```python
from build123d import *

# Parameters (mm, degrees)
SKETCH1_R           = 30
SKETCH1_R_2         = 27.5
BOSS_EXTRUDE1_DEPTH = 100
SKETCH1_2_R         = 27.5
BOSS_EXTRUDE2_DEPTH = 5
SKETCH2_W           = 1.5
SKETCH2_H           = 49.5
BOSS_EXTRUDE3_DEPTH = 40
SKETCH3_W           = 42
SKETCH3_H           = 49.5
BOSS_EXTRUDE4_DEPTH = 2
BOSS_EXTRUDE5_DEPTH = 49.5


with BuildPart() as part:
    # Sketch1 → Boss-Extrude1 (new body)
    with BuildSketch(Plane(origin=(0, 0, 0), x_dir=(1, 0, 0), z_dir=(0, 1, 0))):
        with Locations(Location((0, 0, 0), (0, 0, 270))):
            Circle(SKETCH1_R)
        with Locations(Location((0, 0, 0), (0, 0, 270))):
            Circle(SKETCH1_R_2, mode=Mode.SUBTRACT)
    extrude(amount=BOSS_EXTRUDE1_DEPTH)

    # Sketch1<2> → Boss-Extrude2 (add)
    with BuildSketch(Plane(origin=(0, 0, 0), x_dir=(1, 0, 0), z_dir=(0, 1, 0))):
        with Locations(Location((0, 0, 0), (0, 0, 270))):
            Circle(SKETCH1_2_R)
    extrude(amount=BOSS_EXTRUDE2_DEPTH)

    # Sketch2 → Boss-Extrude3 (add)
    with BuildSketch(Plane.XZ):
        with Locations((-20.25, 0)):
            Rectangle(SKETCH2_W, SKETCH2_H)
        with Locations((20.25, 0)):
            Rectangle(SKETCH2_W, SKETCH2_H)
    extrude(amount=BOSS_EXTRUDE3_DEPTH)

    # Sketch3 → Boss-Extrude4 (add)
    with BuildSketch(Plane.XZ):
        Rectangle(SKETCH3_W, SKETCH3_H)
    extrude(amount=-BOSS_EXTRUDE4_DEPTH)

    # Sketch4 → Boss-Extrude5 (add)
    with BuildSketch(Plane(origin=(0, 0, -24.75), x_dir=(-1, 0, 0), z_dir=(0, 0, -1))):
        Polygon((21, -40), (22.5, -38.5), (21, -38.5), align=None)
        Polygon((-21, -40), (-22.5, -38.5), (-21, -38.5), align=None)
    extrude(amount=-BOSS_EXTRUDE5_DEPTH)


solid = part.part
```
CAD build for the part. Positions are in the model's coordinates, mm. A direction names the side the tool comes from. Give positions to 0.01 mm unless a question says otherwise; leave off trailing zeros. Loops run counter-clockwise (first coordinate to the right, second up) from the corner with the lowest first, then second, coordinate; pieces in that order, holes last. Notation, with made-up numbers: (34.5, 23.5) -> (74.5, 23.5) arc R13 ccw to (74.5, 28.5) -> close; hole circle Ø11 at (-12, 64). An arc over 180 degrees is marked (long way). Use a Markdown table: item, result.
1. Slice it at D-D (z = 0). List the corners of the cut face in (x, y).
Check result:
| item | result |
|---|---|
| outline | (-30, 0) -> (-21, 0) -> (-21, -38.5) -> (-22.5, -38.5) -> (-21, -40) -> (-19.5, -40) -> (-19.5, 0) -> (19.5, 0) -> (19.5, -40) -> (21, -40) -> (22.5, -38.5) -> (21, -38.5) -> (21, 0) -> (30, 0) -> (30, 100) -> (27.5, 100) -> (27.5, 5) -> (-27.5, 5) -> (-27.5, 100) -> (-30, 100) -> close |
2. Flat gauge pins, fed straight in: pin 1 (12 mm diameter, centred on y = -12.5, z = -1, fed in from +X); pin 2 (1 mm diameter, centred on x = 23.5, y = 55, fed in from -Z); pin 3 (10 mm diameter, centred on y = 28.5, z = -7, fed in from -X). Where does each tip first touch, or does it go through?
Check result:
| item | result |
|---|---|
| pin 1 | stops at x = 21 |
| pin 2 | stops at z = -19.26 |
| pin 3 | stops at x = -29.93 |
3. Slice it at B-B (z = 19). List the corners of the cut face in (x, y).
Check result:
| item | result |
|---|---|
| outline | (-23.22, 0) -> (-21, 0) -> (-21, -38.5) -> (-22.5, -38.5) -> (-21, -40) -> (-19.5, -40) -> (-19.5, 0) -> (19.5, 0) -> (19.5, -40) -> (21, -40) -> (22.5, -38.5) -> (21, -38.5) -> (21, 0) -> (23.22, 0) -> (23.22, 100) -> (19.88, 100) -> (19.88, 5) -> (-19.88, 5) -> (-19.88, 100) -> (-23.22, 100) -> close |
4. Slice it at A-A (x = 0). List the corners of the cut face in (y, z), plus the area to 3 significant figures.
Check result:
| item | result |
|---|---|
| outline | (0, -30) -> (100, -30) -> (100, -27.5) -> (5, -27.5) -> (5, 27.5) -> (100, 27.5) -> (100, 30) -> (0, 30) -> close |
| area | 775 mm^2 |
5. Slice it at C-C (y = 26). List the corners of the cut face in (x, z), plus the area to 3 significant figures.
Check result:
| item | result |
|---|---|
| outline | circle Ø60 at (0, 0); hole circle Ø55 at (0, 0) |
| area | 452 mm^2 |
6. Mould opens along Z. For faces 1 (the cylindrical face through (1.32, 49.3, -29.97)), 2 (the flat face through (-20, -17, 24.75)), 3 (the cylindrical face through (-24.397, 51.835, 12.69)) say: pulls with the +Z half, pulls with the -Z half, needs draft (parallel to the pull), parting line crosses it, or undercut.
Check result:
| item | result |
|---|---|
| face 1 | parting line crosses it |
| face 2 | pulls with the +Z half |
| face 3 | undercut |
7. Wall check: L1, parallel to X at y = -32, z = 8.5; L2, parallel to X at y = 69, z = 0. Give the ranges that are in metal, low to high. Write a range as [from, to].
Check result:
| item | result |
|---|---|
| L1 | x = [-21, -19.5], [19.5, 21] |
| L2 | x = [-30, -27.5], [27.5, 30] |
8. Which spindle directions (+Z, -Z, +X, -X, +Y, -Y) get a long thin tool onto all of the face, cutting with end or side? Do faces 4 (the flat face through (19.5, -20, 0)), 5 (the flat face through (-24, 0, 0)), 6 (the flat face through (0, 5, 0)), 7 (the flat face through (20, 2, -24)), 8 (the flat face through (20, 2, 24)). Say none if no direction does.
Check result:
| item | result |
|---|---|
| face 4 | +Z, -Z, -Y |
| face 5 | +Z, -Z, -X |
| face 6 | +Y |
| face 7 | -Z, +X, +Y |
| face 8 | +Z, +X, +Y |
